Source: CAD feature listing. Evaluate the final solid. Frame: model axes, mm. Face numbers are marked on the shaded views. A direction names the side the tool comes from. Give positions to 0.01 mm unless a question says otherwise; leave off trailing zeros. Order: outer loops, then holes, each group sorted by start corner. A loop starts at its lowest first (then second) coordinate and runs counter-clockwise, first axis right, second up.
```python
from build123d import *

# Parameters (mm, degrees)
F1_DEPTH = 270


with BuildPart() as f1:
    # F0 (on Right) → F1 (new body, symmetric)
    with BuildSketch(Plane.YZ):
        Polygon((57.5, 0), (0, 0), (-57.5, 0), (-57.5, 50), (-59.75, 50), (-59.75, 0), (-174.75, 0), (-174.75, 50), (-177, 50), (-177, -5), (0, -5), (177, -5), (177, 50), (174.75, 50), (174.75, 0), (59.75, 0), (59.75, 50), (57.5, 50), align=None)
    extrude(amount=F1_DEPTH, both=True)


solid = f1.part
```
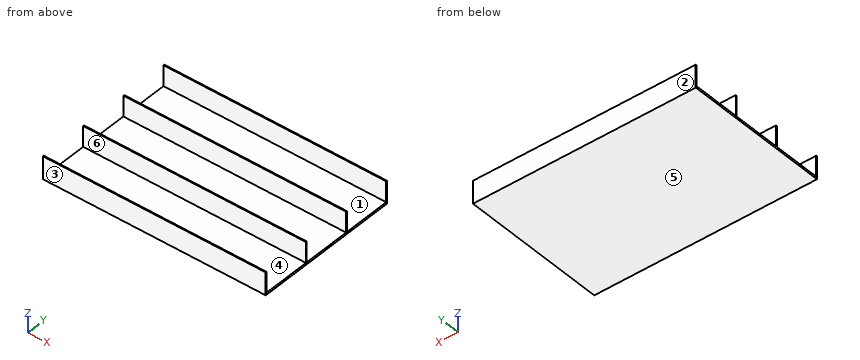
1) Material intervals for L1, parallel to Y at x = 34, z = 22; L2, parallel to Z at x = -24, y = 22, sorted ascending.
Report:
L1: y = -177 to -174.75, -59.75 to -57.5, 57.5 to 59.75, 174.75 to 177
L2: z = -5 to 0
2) Section query A-A, the plane z = 13. Return the cut outline in (x, y).
Report:
outline: (-270, -177) - (270, -177) - (270, -174.75) - (-270, -174.75) - close; (-270, -59.75) - (270, -59.75) - (270, -57.5) - (-270, -57.5) - close; (-270, 57.5) - (270, 57.5) - (270, 59.75) - (-270, 59.75) - close; (-270, 174.75) - (270, 174.75) - (270, 177) - (-270, 177) - close
3) Section query C-C, the plane y = 85. Return the cut outline in (x, z), and give its area (3 significant figures).
Report:
outline: (-270, -5) - (270, -5) - (270, 0) - (-270, 0) - close
area: 2,700 mm2
4) Section query B-B, the plane x = -161.5. Return the cut outline in (y, z).
Report:
outline: (-177, -5) - (177, -5) - (177, 50) - (174.75, 50) - (174.75, 0) - (59.75, 0) - (59.75, 50) - (57.5, 50) - (57.5, 0) - (-57.5, 0) - (-57.5, 50) - (-59.75, 50) - (-59.75, 0) - (-174.75, 0) - (-174.75, 50) - (-177, 50) - close
5) Draft query along Y for the marked faces 3, 4, 5 and 6. Return one class per face: +Y half, -Y half, draft (parallel to the pull), parting line (faces both ways), or undercut.
Report:
face 3: -Y half
face 4: undercut
face 5: draft
face 6: undercut
6) Reachability of the marked faces 1 and 2 from +Z, -Z, +X, -X, +Y, -Y: full face, straight path, thin tool, end or side. Return the list, or none.
Report:
face 1: +Z, +X, -X
face 2: +Z, -Z, +X, -X, +Y
